```python
from build123d import *

# Parameters (mm, degrees)
F0_W     = 98.3195006847
F0_H     = 47.5294552743
F1_DEPTH = 105.156
F2_W     = 98.3195006847
F2_H     = 28.2054126678
F3_DEPTH = 46.482


with BuildPart() as f1:
    # F0 (on Front) → F1 (new body)
    with BuildSketch(Plane.XZ):
        with Locations((-0.6270371377, 23.7647276372)):
            Rectangle(F0_W, F0_H)
    extrude(amount=F1_DEPTH)

    # F2 (on face) → F3 (join)
    with BuildSketch(Plane.XY.offset(47.5294552743)):
        with Locations((-0.6270371377, -91.0532936661)):
            Rectangle(F2_W, F2_H)
    extrude(amount=F3_DEPTH)


solid = f1.part
```
Can you work these out from the model? Positions are in its coordinate system, mm. A direction names the side the tool comes from. Coordinates: 2 decimals unless noted, no trailing zeros. Loops run counter-clockwise (first coordinate to the right, second up) from the corner with the lowest first, then second, coordinate; pieces in that order, holes last. Notation, with made-up numbers: M 31.25,-19.5 L 39.25,-19.5 A16 cw 39.25,4.5 Z; hole C 21.25,87 d3. An arc over 180 degrees is marked long. Put each result on its own line as item: value. Start each with the question number.
(1) Imagine slicing it at B-B on z = 55. List the corners of the cut face in (x, y) for me, and give its area (3 significant figures).
(2) Imagine slicing it at C-C on y = -44.5. List the corners of the cut face in (x, z) for me, and give its area (3 significant figures).
(3) Which directions (+Z, -Z, +X, -X, +Y, -Y) give clear straight access to the entire face, cutting with the end or side of a thin tool? Please do faces 1 (the face through (-1, -38, 47.529)), 2 (the face through (-1, -105.156, 46)).
(4) Will these pins go through, and if not, where does the flat tip stop? pin 1 Ø3 at (x, z) = (32, 64.5) entering from +Y; pin 2 Ø12 at (x, y) = (-10, -66.5) entering from +Z.
(5) Imagine slicing it at A-A on x = 2.5. List the corners of the cut face in (y, z) for me, and give its area (3 significant figures).
(6) I need wall thicknesses on probe 1 along Z at (x, y) = (8, -13); probe 2 along Y at (x, z) = (-41, 67). Which ranges of each line are inside material? Lowest first, please.
Worked answers:
1. outline: M -49.79,-105.16 L 48.53,-105.16 L 48.53,-76.95 L -49.79,-76.95 Z
1. area: 2,770 mm2
2. outline: M -49.79,0 L 48.53,0 L 48.53,47.53 L -49.79,47.53 Z
2. area: 4,670 mm2
3. face 1: +Z, +X, -X, +Y
3. face 2: +Z, -Z, +X, -X, -Y
4. pin 1: stops at y = -76.95
4. pin 2: stops at z = 47.53
5. outline: M -105.16,0 L 0,0 L 0,47.53 L -76.95,47.53 L -76.95,94.01 L -105.16,94.01 Z
5. area: 6,310 mm2
6. probe 1: z = 0 to 47.53
6. probe 2: y = -105.16 to -76.95
